```python
from build123d import *

# Parameters (mm, degrees)
PAD_DEPTH            = 6.5
POCKET_DEPTH         = 6
SKETCH002_R          = 13.5
POCKET001_DEPTH      = 1
SKETCH003_W          = 5.4
SKETCH003_H          = 6.5
PAD001_DEPTH         = 3.5
POCKET002_DEPTH      = 10
SKETCH010_W          = 3.95
SKETCH010_H          = 6.5
PAD002_DEPTH         = 3.5
POCKET005_DEPTH      = 10
SKETCH015_R          = 2.2
SKETCH015_R_2        = 1.025
PAD003_DEPTH         = 2
POCKET009_DEPTH      = 4
POCKET010_DEPTH      = 4
PAD004_DEPTH         = 4
POCKET013_DEPTH      = 12.151
POCKET013_DEPTH_BACK = 36.251
SKETCH022_R          = 0.6
POCKET014_DEPTH      = 2
SKETCH023_R          = 0.6
POCKET015_DEPTH      = 2
SKETCH024_R          = 13.5
PAD005_DEPTH         = 0.5
SKETCH025_R          = 20.45
SKETCH025_R_2        = 19.85
POCKET016_DEPTH      = 0.3
SKETCH026_R          = 1
POCKET017_DEPTH      = 5


with BuildPart() as part:
    # Sketch → Pad (new body)
    with BuildSketch(Plane.XY):
        with BuildLine():
            Line((-22.5019915649, 16), (-22.5019915649, -16))
            Line((-22.5019915649, -16), (-16.2858834578, -17.9))
            ThreePointArc((-16.2858834578, -17.9), (-0.4552796053, -24.1957169863), (15.6009615088, -18.5))
            Line((15.6009615088, -18.5), (24.5395016581, -17.45))
            Line((24.5395016581, 17.45), (24.5395016581, -17.45))
            Line((15.6009615088, 18.5), (24.5395016581, 17.45))
            ThreePointArc((15.6009615088, 18.5), (-0.4552796053, 24.1957169863), (-16.2858834578, 17.9))
            Line((-22.5019915649, 16), (-16.2858834578, 17.9))
        make_face()
    extrude(amount=PAD_DEPTH)

    # Sketch001 → Pocket (cut)
    with BuildSketch(Plane.XY):
        with BuildLine():
            Line((-14.8539557021, 16.9), (-21.2122180433, 15.55))
            Line((-21.2122180433, 15.55), (-21.2122180433, -15.55))
            Line((-21.2122180433, -15.55), (-14.8539557021, -16.9))
            ThreePointArc((-14.8539557021, -16.9), (-0.0760301383, -22.4998715423), (14.739402973, -17))
            Line((14.739402973, -17), (23.6191552218, -16.4))
            Line((23.6191552218, 16.4), (23.6191552218, -16.4))
            Line((14.739402973, 17), (23.6191552218, 16.4))
            ThreePointArc((14.739402973, 17), (-0.0760301383, 22.4998715423), (-14.8539557021, 16.9))
        make_face()
    extrude(amount=POCKET_DEPTH, mode=Mode.SUBTRACT)

    # Sketch002 (on Face19 of Pocket) → Pocket001 (cut)
    with BuildSketch(Plane(origin=(0, 0, 6), x_dir=(1, 0, 0), z_dir=(0, 0, -1))):
        Circle(SKETCH002_R)
    extrude(amount=-POCKET001_DEPTH, mode=Mode.SUBTRACT)

    # Sketch003 (on Face7 of Pad) → Pad001 (join)
    with BuildSketch(Plane.YZ.offset(24.5395016581)):
        with Locations((-14.75, 3.25)):
            Rectangle(SKETCH003_W, SKETCH003_H)
        with Locations((14.75, 3.25)):
            Rectangle(SKETCH003_W, SKETCH003_H)
    extrude(amount=PAD001_DEPTH)

    # Sketch006 (on Face22 of Pad001) → Pocket002 (cut)
    with BuildSketch(Plane.XY.offset(6.5)):
        with BuildLine():
            ThreePointArc((24.5395016581, 17.45), (26.1592830786, 16.2095505764), (28.0395016581, 15.4176006311))
            Line((28.0395016581, 17.45), (28.0395016581, 15.4176006311))
            Line((28.0395016581, 17.45), (24.5395016581, 17.45))
        make_face()
        with BuildLine():
            ThreePointArc((28.0395016581, -15.4176006311), (26.1592830786, -16.2095505765), (24.5395016581, -17.4500000001))
            Line((28.0395016581, -17.45), (24.5395016581, -17.45))
            Line((28.0395016581, -15.4176006311), (28.0395016581, -17.45))
        make_face()
    extrude(amount=-POCKET002_DEPTH, mode=Mode.SUBTRACT)

    # Sketch010 (on Face3 of Pad) → Pad002 (join)
    with BuildSketch(Plane(origin=(-22.5019915649, 0, 0), x_dir=(0, -1, 0), z_dir=(-1, 0, 0))):
        with Locations((-14.025, 3.25)):
            Rectangle(SKETCH010_W, SKETCH010_H)
        with Locations((14.025, 3.25)):
            Rectangle(SKETCH010_W, SKETCH010_H)
    extrude(amount=PAD002_DEPTH)

    # Sketch011 (on Face28 of Pad002) → Pocket005 (cut)
    with BuildSketch(Plane.XY.offset(6.5)):
        Polygon((-26.0019915649, 16), (-22.5019915649, 16), (-26.0019915649, 14.5), align=None)
        Polygon((-22.5019915649, -16), (-26.0019915649, -14.5), (-26.0019915649, -16), align=None)
    extrude(amount=-POCKET005_DEPTH, mode=Mode.SUBTRACT)

    # Sketch015 (on Face19 of Pocket) → Pad003 (join)
    with BuildSketch(Plane(origin=(0, 0, 6), x_dir=(1, 0, 0), z_dir=(0, 0, -1))):
        with Locations((-18.42, 13.32)):
            Circle(SKETCH015_R)
        with Locations((-18.42, 13.32)):
            Circle(SKETCH015_R_2, mode=Mode.SUBTRACT)
        with Locations((7.27, 18.56)):
            Circle(SKETCH015_R)
        with Locations((7.27, 18.56)):
            Circle(SKETCH015_R_2, mode=Mode.SUBTRACT)
        with Locations((5.37, -19.79)):
            Circle(SKETCH015_R)
        with Locations((5.37, -19.79)):
            Circle(SKETCH015_R_2, mode=Mode.SUBTRACT)
        with Locations((-18.42, -13.32)):
            Circle(SKETCH015_R)
        with Locations((-18.42, -13.32)):
            Circle(SKETCH015_R_2, mode=Mode.SUBTRACT)
    extrude(amount=PAD003_DEPTH)

    # Sketch016 (on Face4 of Pocket) → Pocket009 (cut)
    with BuildSketch(Plane(origin=(0, 0, 0), x_dir=(1, 0, 0), z_dir=(0, 0, -1))):
        with BuildLine():
            Line((-4.9992330338, 23.6779996848), (-5.0007669662, 21.9372361465))
            ThreePointArc((5.0007669662, 21.9372361465), (0, 22.5), (-5.0007669662, 21.9372361465))
            Line((5.0007669662, 23.6776757675), (5.0007669662, 21.9372361465))
            ThreePointArc((5.0007669662, 23.6776757675), (0.00078388, 24.1999999873), (-4.9992330338, 23.6779996848))
        make_face()
    extrude(amount=-POCKET009_DEPTH, mode=Mode.SUBTRACT)

    # Sketch017 (on Face4 of Pocket) → Pocket010 (cut)
    with BuildSketch(Plane(origin=(0, 0, 0), x_dir=(1, 0, 0), z_dir=(0, 0, -1))):
        with BuildLine():
            ThreePointArc((-3.2541322314, -22.2634369184), (0, -22.5), (3.2541322314, -22.2634369184))
            Line((3.2541322314, -22.2634369184), (3.5, -23.9455632634))
            ThreePointArc((-3.5, -23.9455632634), (0, -24.2), (3.5, -23.9455632634))
            Line((-3.2541322314, -22.2634369184), (-3.5, -23.9455632634))
        make_face()
        with BuildLine():
            ThreePointArc((-13.9498796389, -17.6536358312), (-11.25, -19.4855715851), (-8.3135572795, -20.9077680626))
            Line((-8.3135572795, -20.9077680626), (-8.9416927184, -22.487466094))
            ThreePointArc((-15.0038705449, -18.987466094), (-12.1, -20.9578147716), (-8.9416927184, -22.487466094))
            Line((-13.9498796389, -17.6536358312), (-15.0038705449, -18.987466094))
        make_face()
        with BuildLine():
            ThreePointArc((8.3135572795, -20.9077680626), (11.25, -19.4855715851), (13.9498796389, -17.6536358312))
            Line((13.9498796389, -17.6536358312), (15.0038705449, -18.987466094))
            ThreePointArc((8.9416927184, -22.487466094), (12.1, -20.9578147716), (15.0038705449, -18.987466094))
            Line((8.3135572795, -20.9077680626), (8.9416927184, -22.487466094))
        make_face()
    extrude(amount=-POCKET010_DEPTH, mode=Mode.SUBTRACT)

    # Sketch018 (on Face8 of Pocket005) → Pad004 (join)
    with BuildSketch(Plane(origin=(0, 0, 0), x_dir=(1, 0, 0), z_dir=(0, 0, -1))):
        Polygon((-26.0019915649, 14.5), (-26.0019915649, 12.05), (-22.5019915649, 12.05), (-22.5019915649, 16), align=None)
        Polygon((-26.0019915649, -12.05), (-22.5019915649, -12.05), (-22.5019915649, -16), (-26.0019915649, -14.5), align=None)
        with BuildLine():
            Line((24.5395016581, 17.4500000001), (24.5395016581, 12.05))
            Line((28.0395016581, 12.05), (24.5395016581, 12.05))
            Line((28.0395016581, 15.4176006311), (28.0395016581, 12.05))
            ThreePointArc((24.5395016581, 17.4500000001), (26.1592830786, 16.2095505765), (28.0395016581, 15.4176006311))
        make_face()
        with BuildLine():
            Line((24.5395016581, -12.05), (24.5395016581, -17.45))
            ThreePointArc((28.0395016581, -15.4176006311), (26.1592830786, -16.2095505764), (24.5395016581, -17.45))
            Line((28.0395016581, -12.05), (28.0395016581, -15.4176006311))
            Line((24.5395016581, -12.05), (28.0395016581, -12.05))
        make_face()
    extrude(amount=PAD004_DEPTH)

    # Sketch021 (on Face50 of Pad004) → Pocket013 (cut, two sides)
    with BuildSketch(Plane(origin=(0, -12.05, 0), x_dir=(-1, 0, 0), z_dir=(0, 1, 0))) as pocket013_sk:
        with BuildLine():
            Line((-24.5395016581, -4), (-24.5395016581, -2))
            ThreePointArc((-26.5395016581, -4), (-25.1252880957, -3.4142135624), (-24.5395016581, -2))
            Line((-24.5395016581, -4), (-26.5395016581, -4))
        make_face()
        with BuildLine():
            Line((22.5019915649, -4), (22.5019915649, -2))
            ThreePointArc((22.5019915649, -2), (23.0877780026, -3.4142135624), (24.5019915649, -4))
            Line((22.5019915649, -4), (24.5019915649, -4))
        make_face()
        with BuildLine():
            Line((-28.0395016581, 0), (-28.0395016581, 6.5))
            Line((-28.0395016581, 6.5), (-24.5395016581, 6.5))
            ThreePointArc((-24.5395016581, 6.5), (-27.1088837932, 3.6912057651), (-28.0395016581, 0))
        make_face()
        with BuildLine():
            Line((26.0019915649, 6.5), (26.0019915649, 0))
            ThreePointArc((26.0019915649, 0), (25.0713737, 3.6912057651), (22.5019915649, 6.5))
            Line((26.0019915649, 6.5), (22.5019915649, 6.5))
        make_face()
    extrude(amount=-POCKET013_DEPTH, mode=Mode.SUBTRACT)
    extrude(pocket013_sk.sketch, amount=POCKET013_DEPTH_BACK, mode=Mode.SUBTRACT)

    # Sketch022 (on Face66 of Pocket013) → Pocket014 (cut)
    with BuildSketch(Plane.XZ.offset(-12.05)):
        with Locations((-24.7019915649, -2.7)):
            Circle(SKETCH022_R)
        with Locations((26.7395016581, -2.7)):
            Circle(SKETCH022_R)
    extrude(amount=-POCKET014_DEPTH, mode=Mode.SUBTRACT)

    # Sketch023 (on Face49 of Pocket014) → Pocket015 (cut)
    with BuildSketch(Plane(origin=(0, -12.05, 0), x_dir=(-1, 0, 0), z_dir=(0, 1, 0))):
        with Locations((-26.7395016581, -2.7)):
            Circle(SKETCH023_R)
        with Locations((24.7019915649, -2.7)):
            Circle(SKETCH023_R)
    extrude(amount=-POCKET015_DEPTH, mode=Mode.SUBTRACT)

    # Sketch024 (on Face16 of Pocket015) → Pad005 (join)
    with BuildSketch(Plane.XY.offset(6.5)):
        with BuildLine():
            ThreePointArc((-22.5019915649, -8.9050758341), (24.2, 0), (-22.5019915649, 8.9050758341))
            Line((-22.5019915649, 8.9050758341), (-22.5019915649, -8.9050758341))
        make_face()
        Circle(SKETCH024_R, mode=Mode.SUBTRACT)
    extrude(amount=PAD005_DEPTH)

    # Sketch025 (on Face42 of Pad005) → Pocket016 (cut)
    with BuildSketch(Plane.XY.offset(7)):
        Circle(SKETCH025_R)
        Circle(SKETCH025_R_2, mode=Mode.SUBTRACT)
    extrude(amount=-POCKET016_DEPTH, mode=Mode.SUBTRACT)

    # Sketch026 (on DatumPlane) → Pocket017 (cut)
    with BuildSketch(Plane.XZ.offset(25)):
        with Locations((-6.5, 4.8)):
            Circle(SKETCH026_R)
    extrude(amount=-POCKET017_DEPTH, mode=Mode.SUBTRACT)


solid = part.part
```
The model under review builds one solid part; all positions refer to its coordinate system, in mm. A direction names the side the tool comes from. Coordinates: 2 decimals unless noted, no trailing zeros. Write each loop counter-clockwise with the first axis right and the second up, starting at its lowest first coordinate (ties: lowest second). Pieces come first, ordered by that corner, then holes.
1) We need section D-D on x = -6.5. State the section outline as (y, z) points.
2) We need section C-C on y = 10. State the section outline as (x, z) points, then the cut area to 3 significant figures.
3) The part is to be moulded in two halves that separate along Y. For faces 6 (the face through (0, -23, 4)), 7 (the face through (8.29, -16.61, 5.01)), 8 (the face through (8, -20, 4)), 9 (the face through (-19.437, -16.937, 3.204)), say which applies: pulls with the +Y half, pulls with the -Y half, needs draft (parallel to the pull), parting line crosses it, or undercut.
4) Machinability: for faces 1 (the face through (-17, 11, 6.7)), 2 (the face through (-8.623, 21.687, 1.972)), 3 (the face through (-3.375, 23.093, 1.972)), 4 (the face through (24.54, 15, -1)), 5 (the face through (24.1, -4, 6.5)), which of the approach directions +Z, -Z, +X, -X, +Y, -Y give a long, thin tool a straight path to every point of the face, cutting with its end or side? Answer none if there is none.
5) To check wall thickness, follow probe 1 along X at (y, z) = (-6, 4.75); probe 2 along X at (y, z) = (-20, 4.5); probe 3 along X at (y, z) = (-13.32, 4.8) (3 decimals). State the ranges of each line that lie inside material, in increasing order.
6) We need section B-B on x = 0. State the section outline as (y, z) points.
7) Clearance check with flat-ended pins moving along their axes: pin 1 Ø5 at (y, z) = (-15, 0.5) entering from -X; pin 2 Ø3 at (x, z) = (26, 2.5) entering from -Y; pin 3 Ø6 at (x, z) = (-7.5, 0.5) entering from +Y; pin 4 Ø0.7 at (x, z) = (-24.7, -2.7) entering from -Y. State where each tip first meets the part, or that it passes through.
8) We need section A-A on z = -1. State the section outline as (x, y) points, then the cut area to 3 significant figures.
Answer list:
1. outline: (-23.31, 0) - (-21.54, 0) - (-21.54, 3.8) - (-23.31, 3.8) - close; (-23.31, 5.8) - (-21.54, 5.8) - (-21.54, 6) - (-11.83, 6) - (-11.83, 7) - (-18.76, 7) - (-18.76, 6.7) - (-19.39, 6.7) - (-19.39, 7) - (-23.31, 7) - close; (11.83, 6) - (21.54, 6) - (21.54, 0) - (23.31, 0) - (23.31, 7) - (19.39, 7) - (19.39, 6.7) - (18.76, 6.7) - (18.76, 7) - (11.83, 7) - close
2. outline: (-22.5, 0) - (-21.21, 0) - (-21.21, 6) - (-9.07, 6) - (-9.07, 7) - (-17.15, 7) - (-17.15, 6.7) - (-17.84, 6.7) - (-17.84, 7) - (-22.04, 7) - (-22.04, 6.5) - (-22.5, 6.5) - close; (9.07, 6) - (23.62, 6) - (23.62, 0) - (24.54, 0) - (24.54, 6.5) - (22.04, 6.5) - (22.04, 7) - (17.84, 7) - (17.84, 6.7) - (17.15, 6.7) - (17.15, 7) - (9.07, 7) - close
2. area: 40.3 mm2
3. face 6: needs draft
3. face 7: undercut
3. face 8: undercut
3. face 9: pulls with the -Y half
4. face 1: +Z
4. face 2: -Z, -X
4. face 3: -Z, +Y
4. face 4: -Z, +Y, -Y
4. face 5: +Z, +X
5. probe 1: x = -22.5 to -21.21, 23.62 to 24.54
5. probe 2: x = -13.62 to -10.31, 5.61 to 8.93, 10.31 to 13.62
5. probe 3: x = -24.346 to -21.212, -20.62 to -19.445, -17.395 to -16.22, 23.619 to 26.384
6. outline: (-24.2, 4) - (-22.5, 4) - (-22.5, 6) - (-13.5, 6) - (-13.5, 7) - (-19.85, 7) - (-19.85, 6.7) - (-20.45, 6.7) - (-20.45, 7) - (-24.2, 7) - close; (13.5, 6) - (22.5, 6) - (22.5, 4) - (24.2, 4) - (24.2, 7) - (20.45, 7) - (20.45, 6.7) - (19.85, 6.7) - (19.85, 7) - (13.5, 7) - close
7. pin 1: stops at x = -26
7. pin 2: stops at y = -17.45
7. pin 3: stops at y = 23.78
7. pin 4: stops at y = -15.21
8. outline: (-26, -14.5) - (-22.5, -16) - (-22.5, -12.05) - (-26, -12.05) - close; (-26, 12.05) - (-22.5, 12.05) - (-22.5, 16) - (-26, 14.5) - close; (24.54, -17.45) arc R8.03 cw to (28.04, -15.42) - (28.04, -12.05) - (24.54, -12.05) - close; (24.54, 12.05) - (28.04, 12.05) - (28.04, 15.42) arc R8.03 cw to (24.54, 17.45) - close
8. area: 51.7 mm2
